Here's how the part is built. I have some questions about the finished solid (model axes, mm). Face numbers are marked on the shaded views. A direction names the side the tool comes from. Coordinates: 2 decimals unless noted, no trailing zeros. Loops run counter-clockwise (first coordinate to the right, second up) from the corner with the lowest first, then second, coordinate; pieces in that order, holes last. Notation, with made-up numbers: (-16, 84) -> (3, 84) arc R33 cw to (3, 112) -> close; hole circle Ø2 at (-40, 61.25). An arc over 180 degrees is marked (long way). Answer as a JSON object with one key per item and string values. Group by question number.
Q1. I need wall thicknesses on line 1 (Y direction, x = -14, z = 1); line 2 (Y direction, x = 0, z = -1.5); line 3 (Y direction, x = -2, z = 3.75). Which ranges of each line are inside material? Lowest first, please.
Q2. I want a section at A-A on y = 0. Write out the boundary of the cut face in (x, z), then the cut area to 3 significant figures.
Q3. I want a section at C-C on z = 3.5. Write out the boundary of the cut face in (x, y).
Q4. On a 3-axis mill with a long thin cutter (end or side, diameter ignored), from which of +Z, -Z, +X, -X, +Y, -Y can I reach the whole of each face in a straight line? I mean the marked faces 4 and 5. Say none if no direction works.
Q5. Thinking about a two-plate mould opening in X: for the marked faces 1, 2 and 3, which applies, released by +X, released by -X, zero draft, split by the parting line, or undercut?
Q6. I'm going to push flat-ended pins straight in: pin 1 (10.5 mm diameter, centred on x = 0, y = 0, fed in from +Z); pin 2 (6 mm diameter, centred on y = -2, z = -3.5, fed in from +X); pin 3 (4 mm diameter, centred on y = 15, z = 0, fed in from -X); pin 4 (1 mm diameter, centred on y = 23, z = -1.5, fed in from -X). Where does each tip first touch, or does it pass through?
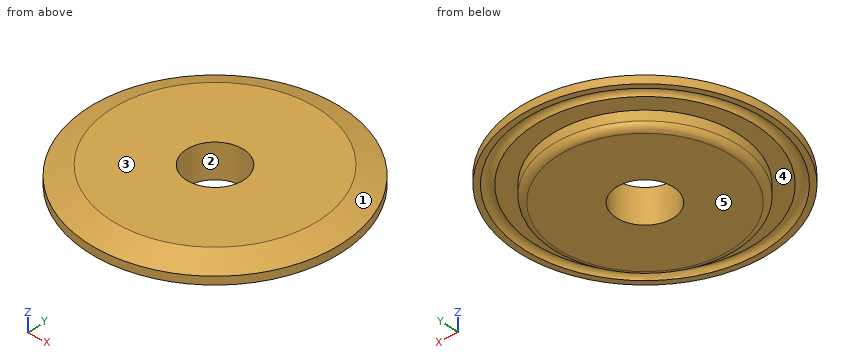
```python
from build123d import *

# Parameters (mm, degrees)
F0_R     = 38.7
F1_DEPTH = 5.45
F2_R     = 28.6
F3_DEPTH = 5
F4_SIZE2 = 3
F4_SIZE  = 7
F5_R     = 2
F12_D    = 17.4625


with BuildPart() as f1:
    # F0 (on Top) → F1 (new body)
    with BuildSketch(Plane.XY):
        Circle(F0_R)
    extrude(amount=F1_DEPTH)

    # F2 (on face) → F3 (join)
    with BuildSketch(Plane(origin=(0, 0, 0), x_dir=(1, 0, 0), z_dir=(0, 0, -1))):
        Circle(F2_R)
    extrude(amount=F3_DEPTH)

    # F4
    f4_edges = [f1.edges().sort_by_distance(p)[0] for p in [
        (-38.7, 0, 5.45),
    ]]
    f4_side = f1.faces().sort_by_distance((0, 0, 5.45))[0]
    chamfer(f4_edges, length=F4_SIZE, length2=F4_SIZE2, reference=f4_side)

    # F5
    f5_edges = [f1.edges().sort_by_distance(p)[0] for p in [
        (-28.6, 0, -5),
    ]]
    fillet(f5_edges, radius=F5_R)

    # F9 (on 3pt) → F11 (revolve, cut)
    with BuildSketch(Plane(origin=(0, 0, 0), x_dir=(0, -1, 0), z_dir=(-1, 0, 0))):
        with BuildLine():
            Line((33.8, 0), (37, 0))
            ThreePointArc((37, 0), (35.4, 1.2468871126), (33.8, 0))
        make_face()
    revolve(axis=Axis((0, 0, 7.6663349755), (0, 0, -1)), mode=Mode.SUBTRACT)

    # F12 (through all)
    with Locations(Plane(origin=(0, 0, -5), x_dir=(1, 0, 0), z_dir=(0, 0, -1))):
        with Locations((0, 0)):
            Hole(F12_D / 2)


solid = f1.part
```
Result set:
{
 "1": {"line 1": "y = -36.08 to -33.46, -31.57 to 31.57, 33.46 to 36.08", "line 2": "y = -28.6 to -8.73, 8.73 to 28.6", "line 3": "y = -35.61 to -8.5, 8.5 to 35.61"},
 "2": {"outline": "(-38.7, 0) -> (-37, 0) arc R1.65 cw to (-33.8, 0) -> (-28.6, 0) -> (-28.6, -3) arc R2 ccw to (-26.6, -5) -> (-8.73, -5) -> (-8.73, 5.45) -> (-31.7, 5.45) -> (-38.7, 2.45) -> close; (8.73, -5) -> (26.6, -5) arc R2 ccw to (28.6, -3) -> (28.6, 0) -> (33.8, 0) arc R1.65 cw to (37, 0) -> (38.7, 0) -> (38.7, 2.45) -> (31.7, 5.45) -> (8.73, 5.45) -> close", "area": "497 mm²"},
 "3": {"outline": "circle Ø72.5 at (0, 0); hole circle Ø17.46 at (0, 0)"},
 "4": {"face 4": "-Z", "face 5": "-Z, +X, -X, +Y, -Y"},
 "5": {"face 1": "split by the parting line", "face 2": "undercut", "face 3": "zero draft"},
 "6": {"pin 1": "passes through", "pin 2": "stops at x = 28.6", "pin 3": "stops at x = -36.45", "pin 4": "stops at x = -17.66"}
}
